Design review of the part built by this model. Coordinates are the model's own, in mm. Round coordinates to 2 decimals unless told otherwise and drop trailing zeros. Order: outer loops, then holes, each group sorted by start corner. A loop starts at its lowest first (then second) coordinate and runs counter-clockwise, first axis right, second up. Notation, with made-up numbers: M 5,55.5 L 26,55.5 A19 cw 26,76.5 Z; hole C 19.5,-38.75 d2. An arc over 180 degrees is marked long. Use a Markdown table: item, result. Add a question column.
(1) Take a section at A-A (x = -25). Write out the cut boundary in (y, z), then the cut area to 3 significant figures.
(2) Take a section at B-B (y = 0.8). Write out the cut boundary in (x, z), then the cut area to 3 significant figures.
(3) To check wall thickness, follow probe 1 along X at (y, z) = (1.1, 0); probe 2 along X at (y, z) = (0.5, 2.5); probe 3 along X at (y, z) = (2.8, 6.5). State the ranges of each line that lie inside material, in increasing order. Write a range as from..to.
(4) Take a section at D-D (z = -9). Write out the cut boundary in (x, y), then the cut area to 3 significant figures.
(5) Take a section at C-C (x = 22). Write out the cut boundary in (y, z), then the cut area to 3 significant figures.
(6) For pin 1 (5 mm diameter, centred on x = 25, z = 0, fed in from -Y), flat-tipped, find the tip position at first contact; note if it passes through.
(7) The part is to be moulded in two halves that separate along Z. For faces 1 (the face through (-26.2, 1.5, -1.6)), 2 (the face through (7, 1, 14)), 3 (the face through (-40, 2, 0)), 4 (the face through (-1, 0, 0)), say which applies: released by +Z, released by -Z, zero draft, split by the parting line, or undercut.
```python
from build123d import *

# Parameters (mm, degrees)
SKETCH_1_W      = 80
SKETCH_1_H      = 28
SKETCH_1_R      = 4.25
SKETCH_1_R_2    = 2
EXTRUDE_1_DEPTH = 3
FILLET_1_RADIUS = 14
FILLET_1_LENGTH = 3


with BuildPart() as part:
    # 草图1 → 凸台-拉伸1 (new body)
    with BuildSketch(Plane(origin=(0, 0, 0), x_dir=(1, 0, 0), z_dir=(0, 1, 0))):
        Rectangle(SKETCH_1_W, SKETCH_1_H)
        with Locations(Location((25, 0, 0), (0, 0, 270))):
            Circle(SKETCH_1_R, mode=Mode.SUBTRACT)
        with Locations(Location((-25, 0, 0), (0, 0, 270))):
            Circle(SKETCH_1_R_2, mode=Mode.SUBTRACT)
    extrude(amount=EXTRUDE_1_DEPTH)

    # 圆角1: full round fillet: the end face becomes a half cylinder, R = half its width
    fillet_1_face = Plane((-40, 1.5, 0), x_dir=(0, 1, 0), z_dir=(-1, 0, 0))  # on the end face: x along it, z out of the body
    fillet_1_slab = fillet_1_face.offset(-FILLET_1_RADIUS / 2) * Box(FILLET_1_LENGTH, 2 * FILLET_1_RADIUS, FILLET_1_RADIUS, mode=Mode.PRIVATE)  # the body's end, R deep
    fillet_1_round = Plane((-26, 1.5, 0), x_dir=(-1, 0, 0), z_dir=(0, 1, 0)) * Cylinder(FILLET_1_RADIUS, FILLET_1_LENGTH, mode=Mode.PRIVATE)  # its axis R under the face
    add(fillet_1_slab - fillet_1_round, mode=Mode.SUBTRACT)


solid = part.part
```
Verdict:
| question | item | result |
|---|---|---|
| 1 | outline | M 0,-14 L 3,-14 L 3,-2 L 0,-2 Z; M 0,2 L 3,2 L 3,14 L 0,14 Z |
| 1 | area | 72.0 mm^2 |
| 2 | outline | M -26,-14 L 40,-14 L 40,14 L -26,14 A14 ccw Z; hole C -25,0 d4; hole C 25,0 d8.5 |
| 2 | area | 2,090 mm^2 |
| 3 | probe 1 | x = -40..-27, -23..20.75, 29.25..40 |
| 3 | probe 2 | x = -39.77..21.56, 28.44..40 |
| 3 | probe 3 | x = -38.4..40 |
| 4 | outline | M -36.72,0 L 40,0 L 40,3 L -36.72,3 Z |
| 4 | area | 230 mm^2 |
| 5 | outline | M 0,-14 L 3,-14 L 3,-3.01 L 0,-3.01 Z; M 0,3.01 L 3,3.01 L 3,14 L 0,14 Z |
| 5 | area | 65.9 mm^2 |
| 6 | pin 1 | passes through |
| 7 | face 1 | undercut |
| 7 | face 2 | released by +Z |
| 7 | face 3 | split by the parting line |
| 7 | face 4 | zero draft |
